Design review of the part built by this model. Coordinates are the model's own, in mm. Face numbers are marked on the shaded views. Give positions to 0.01 mm unless a question says otherwise; leave off trailing zeros. Write each loop counter-clockwise with the first axis right and the second up, starting at its lowest first coordinate (ties: lowest second). Pieces come first, ordered by that corner, then holes. Notation, with made-up numbers: (58, 12.5) -> (87, 12.5) arc R5 ccw to (87, 21.5) -> close; hole circle Ø5 at (88.5, 51). An arc over 180 degrees is marked (long way). Answer as a JSON object with one key per item and string values.
```python
from build123d import *

# Parameters (mm, degrees)
F2_R      = 12.9286
F3_DEPTH  = 12.6238
F3_FACE_R = 12.9286
F0_R      = 11.43
F5_R      = 9.3472
F6_DEPTH  = 36.831


with BuildPart() as f3:
    # F2 (on offset) → F3 (new body)
    with BuildSketch(Plane.YZ.offset(-24.2062)):
        Circle(F2_R)
    extrude(amount=-F3_DEPTH)

    # F3_face (on face) → F4 section 0
    with BuildSketch(Plane.YZ.offset(-24.2062)):
        Circle(F3_FACE_R)
    # F0 (on Right) → F4 section 1
    with BuildSketch(Plane.YZ):
        Circle(F0_R)
    loft()

    # F5 (on face) → F6 (cut, through all)
    with BuildSketch(Plane.YZ):
        Circle(F5_R)
    extrude(amount=-F6_DEPTH, mode=Mode.SUBTRACT)


solid = f3.part
```
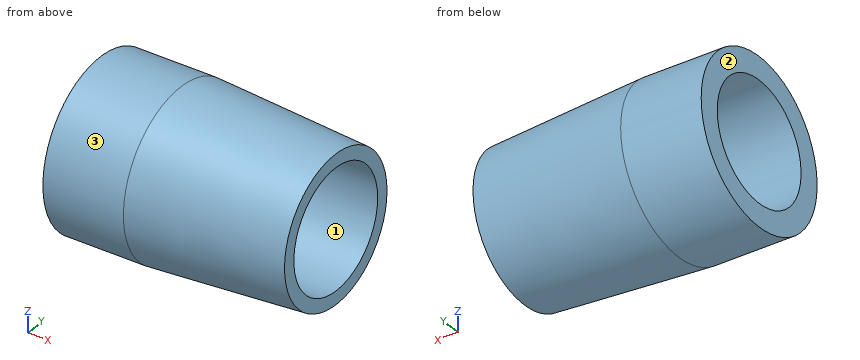
(1) We need section B-B, the plane x = -33.5. State the section outline as (y, z) points, then the cut area to 3 significant figures.
Here are the results:
{"outline": "circle Ø25.86 at (0, 0); hole circle Ø18.69 at (0, 0)", "area": "251 mm²"}
(2) Clearance check with flat-ended pins moving along their axes: pin 1 (10 mm diameter, centred on x = -25.5, z = -10, fed in from +Y); pin 2 (2 mm diameter, centred on x = -30, z = 2.5, fed in from +Y); pin 3 (1.5 mm diameter, centred on x = -20.5, z = 5, fed in from -Y). State where each tip first meets the part, or that it passes through.
Here are the results:
{"pin 1": "stops at y = 11.92", "pin 2": "stops at y = 12.84", "pin 3": "stops at y = -11.97"}
(3) For line 1 along Z through (x, y) = (-8.5, 3.25); line 2 along Z through (x, y) = (-21, 0); line 3 along Y through (x, z) = (-18, -7), list the stretches that pass through material, from the lowest coordinate up.
Here are the results:
{"line 1": "z = -11.51 to -8.76, 8.76 to 11.51", "line 2": "z = -12.73 to -9.35, 9.35 to 12.73", "line 3": "y = -10.41 to -6.19, 6.19 to 10.41"}
(4) We need section A-A, the plane y = 0. State the section outline as (x, z) points.
Here are the results:
{"outline": "(-36.83, -12.93) -> (-24.21, -12.93) -> (0, -11.43) -> (0, -9.35) -> (-36.83, -9.35) -> close; (-36.83, 9.35) -> (0, 9.35) -> (0, 11.43) -> (-24.21, 12.93) -> (-36.83, 12.93) -> close"}
(5) The part is to be moulded in two halves that separate along Z. For the marked faces 1, 2 and 3, say which applies: +Z half, -Z half, draft (parallel to the pull), parting line (faces both ways), or undercut.
Here are the results:
{"face 1": "undercut", "face 2": "draft", "face 3": "parting line"}
(6) We need section C-C, the plane x = -22. State the section outline as (y, z) points.
Here are the results:
{"outline": "circle Ø25.58 at (0, 0); hole circle Ø18.69 at (0, 0)"}
